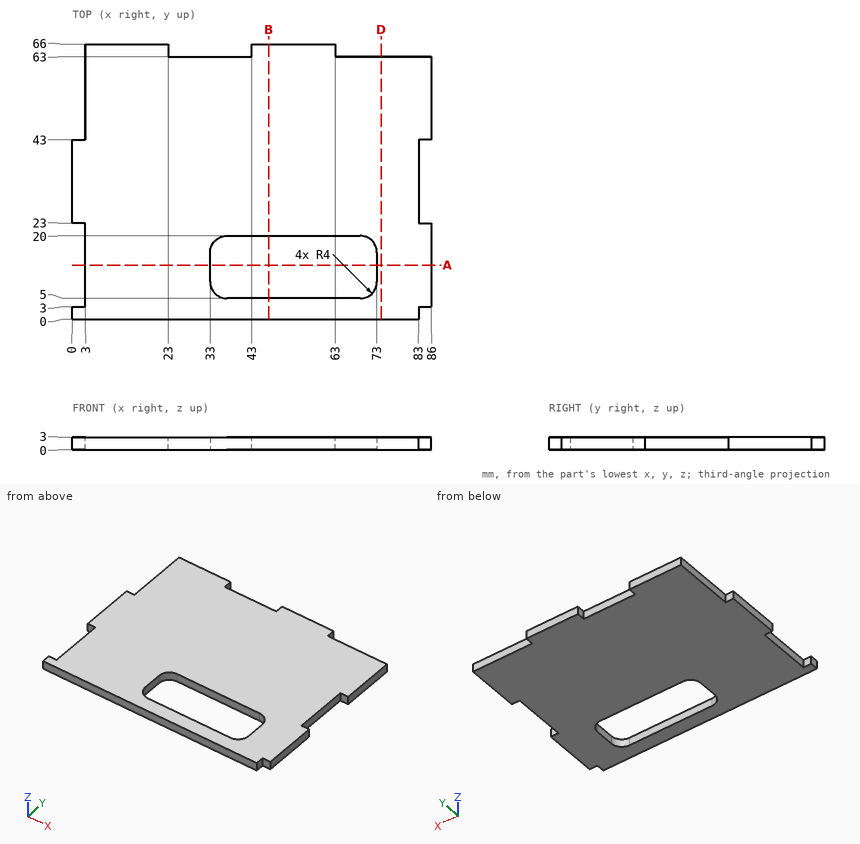
Geometry check sheet. Reference: drawing and pictorial views, mm from the part's lowest x, y, z. Coordinates: 2 decimals unless noted, no trailing zeros. Loops run counter-clockwise (first coordinate to the right, second up) from the corner with the lowest first, then second, coordinate; pieces in that order, holes last. Notation, with made-up numbers: (76, 37.25) - (95, 37.25) arc R22 cw to (95, 55.25) - close; hole circle Ø2 at (-37, -8.5). An arc over 180 degrees is marked (long way). Return JSON: item names as keys, results as strings.
1. Section check B-B, the plane x = 47. Record the boundary of the cut face in (y, z).
Established:
{"outline": "(0, 0) - (5, 0) - (5, 3) - (0, 3) - close; (20, 0) - (66, 0) - (66, 3) - (20, 3) - close"}
2. Go/stop test with flat-tipped pins: pin 1 (0.9 mm diameter, centred on y = 65, z = 1, fed in from +X); pin 2 (0.9 mm diameter, centred on x = 1, z = 1.5, fed in from +Y); pin 3 (0.9 mm diameter, centred on y = 59, z = 1.5, fed in from -X). Record where each tip stops, or that it passes through.
Established:
{"pin 1": "stops at x = 63", "pin 2": "stops at y = 43", "pin 3": "stops at x = 3"}
3. Section check A-A, the plane y = 13. Record the boundary of the cut face in (x, z).
Established:
{"outline": "(3, 0) - (33, 0) - (33, 3) - (3, 3) - close; (73, 0) - (86, 0) - (86, 3) - (73, 3) - close"}
4. Thickness scan on L1, parallel to Y at x = 60.5, z = 1.95; L2, parallel to Y at x = 69, z = 1.65; L3, parallel to X at y = 50, z = 1.3. Record the ranges inside material, lowest first.
Established:
{"L1": "y = 0 to 5, 20 to 66", "L2": "y = 0 to 5, 20 to 63", "L3": "x = 3 to 86"}
5. Section check D-D, the plane x = 74. Record the boundary of the cut face in (y, z).
Established:
{"outline": "(0, 0) - (63, 0) - (63, 3) - (0, 3) - close"}
